Source: three-view drawing plus pictorial views. Frame: mm from the lowest corner of the part. Give positions to 0.01 mm unless a question says otherwise; leave off trailing zeros. Loops run counter-clockwise (first coordinate to the right, second up) from the corner with the lowest first, then second, coordinate; pieces in that order, holes last. Notation, with made-up numbers: M -13.75,26.25 L 15.25,26.25 A7 ccw 15.25,31.25 Z; hole C 11,-9 d9. An arc over 180 degrees is marked long. Write item = value, one per line.
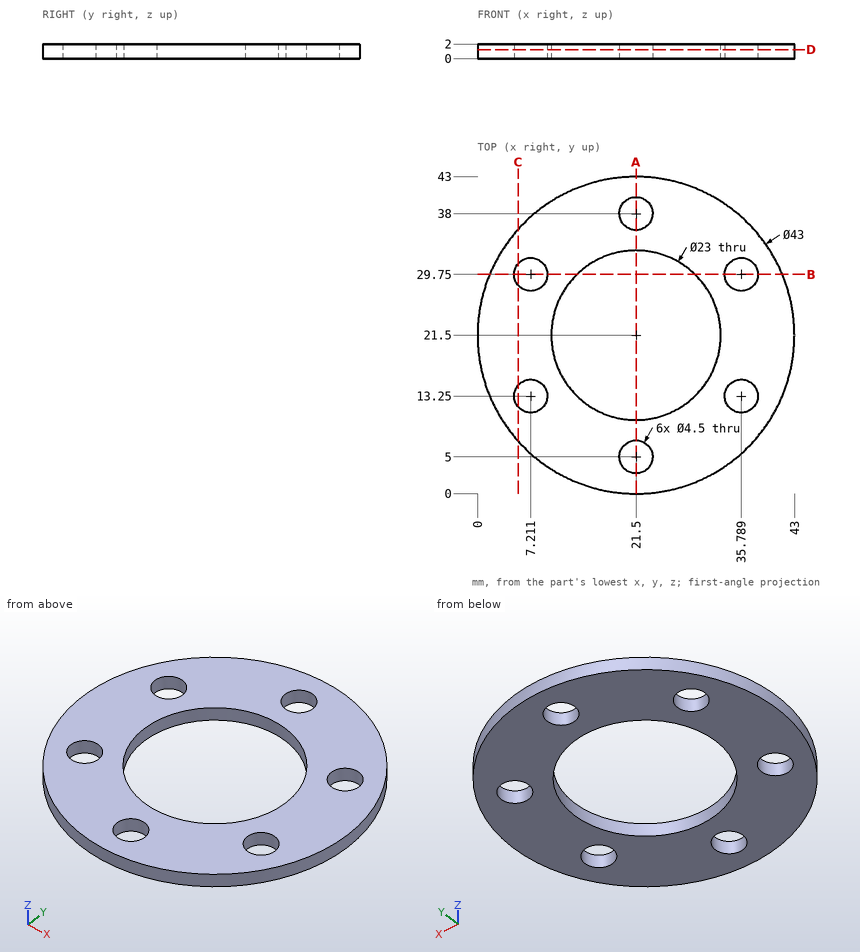
1. Cut plane B-B, the plane y = 29.75. Return the cut outline in (x, z).
Derived:
outline = M 1.65,0 L 4.96,0 L 4.96,2 L 1.65,2 Z; M 9.46,0 L 13.49,0 L 13.49,2 L 9.46,2 Z; M 29.51,0 L 33.54,0 L 33.54,2 L 29.51,2 Z; M 38.04,0 L 41.35,0 L 41.35,2 L 38.04,2 Z
2. Cut plane A-A, the plane x = 21.5. Return the cut outline in (y, z).
Derived:
outline = M 0,0 L 2.75,0 L 2.75,2 L 0,2 Z; M 7.25,0 L 10,0 L 10,2 L 7.25,2 Z; M 33,0 L 35.75,0 L 35.75,2 L 33,2 Z; M 40.25,0 L 43,0 L 43,2 L 40.25,2 Z
3. First-contact query: pin 1 Ø6 at (x, y) = (7.21, 13.25) entering from +Z. Flat tip, straight axial feed; report the tip coordinate or a pass-through.
Derived:
pin_1 = 2
4. Material intervals for probe 1 along Y at (x, z) = (21.5, 1.6); probe 2 along X at (y, z) = (29.75, 0.5) (1 decimal); probe 3 along Y at (x, z) = (34, 1.35) (1 decimal), sorted ascending. Write a range as from..to.
Derived:
probe_1 = 0..2.75, 7.25..10, 33..35.75, 40.25..43
probe_2 = 1.6..5, 9.5..13.5, 29.5..33.5, 38..41.4
probe_3 = 4..11.9, 14.6..28.4, 31.1..39
5. Cut plane C-C, the plane x = 5.5. Return the cut outline in (y, z).
Derived:
outline = M 7.14,0 L 11.79,0 L 11.79,2 L 7.14,2 Z; M 14.71,0 L 28.29,0 L 28.29,2 L 14.71,2 Z; M 31.21,0 L 35.86,0 L 35.86,2 L 31.21,2 Z
6. Cut plane D-D, the plane z = 1.25. Return the cut outline in (x, y).
Derived:
outline = C 21.5,21.5 d43; hole C 7.21,13.25 d4.5; hole C 7.21,29.75 d4.5; hole C 21.5,21.5 d23; hole C 21.5,5 d4.5; hole C 21.5,38 d4.5; hole C 35.79,13.25 d4.5; hole C 35.79,29.75 d4.5
